Geometry check sheet. Reference: the model listing, model coordinates, mm. A direction names the side the tool comes from. Coordinates: 2 decimals unless noted, no trailing zeros. Order: outer loops, then holes, each group sorted by start corner. A loop starts at its lowest first (then second) coordinate and runs counter-clockwise, first axis right, second up. Notation, with made-up numbers: (-7, -29) - (-3, -29) arc R20 cw to (-3, -20) - close; hole circle Ø8 at (60, 85). An arc over 180 degrees is marked (long way). Return JSON: item names as keys, results as strings. Group by question number.
Item 1: Gauge pin test, flat end, axial feed: pin 1 (2 mm diameter, centred on y = 2, z = 6, fed in from +X). Record the tip position at first contact, or that the pin passes through.
Item 2: Section check C-C on y = 4.25. Enter the section's corners in (x, z).
Item 3: Scan lines: probe 1 along X at (y, z) = (2.25, 0.75); probe 2 along Y at (x, z) = (1.75, 6.5); probe 3 along X at (y, z) = (7.5, 7.5). Record each from-to range of solid material in increasing order.
Item 4: Section check D-D on x = 5.25. Enter the section's corners in (y, z), then the cut area to 3 significant figures.
Item 5: Draft check along X on faces 1 (the flat face through (4, 4, 8)), 2 (the flat face through (0, 4.4, 3.6)), 3 (the flat face through (5, 3, 2)). Enter one of: pulls with the +X half, pulls with the -X half, needs draft (parallel to the pull), parting line crosses it, or undercut.
Item 6: Section check B-B on z = 1.75. Enter the section's corners in (x, y).
Item 7: Section check A-A on y = 2. Enter the section's corners in (x, z), then the cut area to 3 significant figures.
Item 8: Tool access check on faces 4 (the flat face through (10, 5, 1)), 5 (the flat face through (7, 1, 1)), 6 (the flat face through (5, 4, 3)), 7 (the flat face through (2, 4, 9)), 8 (the flat face through (2, 3, 6.6)). Record the directions out of +Z, -Z, +X, -X, +Y, -Y that give a thin tool (end or side, any length) a straight path to the whole face; none if there is none.
from build123d import *

# Parameters (mm, degrees)
F1_DEPTH = 9
F2_DEPTH = 6
F3_DEPTH = 3


with BuildPart() as f1:
    # F0 (on Front) → F1 (new body)
    with BuildSketch(Plane.XZ):
        Polygon((0, 4), (0, 0), (4, 0), (4, 3.2), align=None)
        Polygon((7, 2.6), (7, 0), (10, 0), (10, 2), align=None)
        Polygon((0, 9), (0, 7), (4, 6.2), (4, 9), align=None)
        Polygon((4, 3.2), (4, 0), (7, 0), (7, 2.6), align=None)
        Polygon((0, 7), (0, 4), (4, 3.2), (7, 2.6), (10, 2), (10, 5), (4, 6.2), align=None)
    extrude(amount=-F1_DEPTH)

    # F0 (on Front) → F2 (cut)
    with BuildSketch(Plane.XZ):
        Polygon((0, 7), (0, 4), (4, 3.2), (7, 2.6), (10, 2), (10, 5), (4, 6.2), align=None)
    extrude(amount=-F2_DEPTH, mode=Mode.SUBTRACT)

    # F0 (on Front) → F3 (cut)
    with BuildSketch(Plane.XZ):
        Polygon((4, 3.2), (4, 0), (7, 0), (7, 2.6), align=None)
    extrude(amount=-F3_DEPTH, mode=Mode.SUBTRACT)


solid = f1.part
Computed:
{
 "1": {"pin 1": "stops at x = 4"},
 "2": {"outline": "(0, 0) - (10, 0) - (10, 2) - (0, 4) - close; (0, 7) - (4, 6.2) - (4, 9) - (0, 9) - close"},
 "3": {"probe 1": "x = 0 to 4, 7 to 10", "probe 2": "y = 6 to 9", "probe 3": "x = 0 to 4"},
 "4": {"outline": "(3, 0) - (9, 0) - (9, 5.95) - (6, 5.95) - (6, 2.95) - (3, 2.95) - close", "area": "26.7 mm²"},
 "5": {"face 1": "pulls with the +X half", "face 2": "pulls with the -X half", "face 3": "undercut"},
 "6": {"outline": "(0, 0) - (4, 0) - (4, 3) - (7, 3) - (7, 0) - (10, 0) - (10, 9) - (0, 9) - close"},
 "7": {"outline": "(0, 0) - (4, 0) - (4, 3.2) - (0, 4) - close; (0, 7) - (4, 6.2) - (4, 9) - (0, 9) - close; (7, 0) - (10, 0) - (10, 2) - (7, 2.6) - close", "area": "30.9 mm²"},
 "8": {"face 4": "+Z, -Z, +X, +Y, -Y", "face 5": "+Z, -Z, -Y", "face 6": "+X, -Y", "face 7": "+Z, +X, -X, +Y, -Y", "face 8": "-X, -Y"}
}
